from build123d import *
from build123d.topology import SkipClean

# Parameters (mm, degrees)
BOSS_EXTRUDE1_DEPTH      = 3
SKETCH2_W                = 25
SKETCH2_H                = 2
BOSS_EXTRUDE2_DEPTH      = 40
SKETCH3_R                = 0.625
CUT_EXTRUDE1_DEPTH       = 3
SKETCH4_R                = 0.625
CUT_EXTRUDE2_DEPTH       = 3
SKETCH5_W                = 3
SKETCH5_H                = 25
BOSS_EXTRUDE3_DEPTH      = 40
SKETCH7_W                = 19.5
SKETCH7_H                = 75
CUT_EXTRUDE5_DEPTH       = 40
SKETCH10_W               = 25
SKETCH10_H               = 3
BOSS_EXTRUDE4_DEPTH      = 10
SKETCH11_W               = 25
SKETCH11_H               = 3
BOSS_EXTRUDE5_DEPTH      = 10
SKETCH12_W               = 3
SKETCH12_H               = 25
BOSS_EXTRUDE6_DEPTH      = 10
SKETCH13_W               = 3
SKETCH13_H               = 25
BOSS_EXTRUDE7_DEPTH      = 10
SKETCH14_W               = 43
SKETCH14_H               = 35.95813892
BOSS_EXTRUDE11_DEPTH     = 3
SKETCH15_W               = 43
SKETCH15_H               = 35.95813892
BOSS_EXTRUDE12_DEPTH     = 3
SKETCH16_W               = 23
SKETCH16_H               = 28
CUT_EXTRUDE6_DEPTH       = 13
CUT_EXTRUDE7_DEPTH       = 74.054773971
CUT_EXTRUDE7_DEPTH_BACK  = 74.054773971
SKETCH6_R                = 1.625
SKETCH6_R_2              = 3
FILLET1_R                = 10
FILLET2_R                = 10
SKETCH17_W               = 3
SKETCH17_H               = 2.5
CUT_EXTRUDE8_DEPTH       = 30
SKETCH19_W               = 28
SKETCH19_H               = 32
CUT_EXTRUDE9_DEPTH       = 40
CUT_EXTRUDE11_DEPTH      = 60.949979149
CUT_EXTRUDE11_DEPTH_BACK = 60.949979149
SKETCH20_W               = 25.25
SKETCH20_H               = 11.847644437
SKETCH20_W_2             = 25
SKETCH20_H_2             = 13.837487399
CUT_EXTRUDE12_DEPTH      = 70.835521048
CUT_EXTRUDE12_DEPTH_BACK = 70.835521048
CUT_EXTRUDE13_DEPTH      = 56.982140009
CUT_EXTRUDE13_DEPTH_BACK = 56.982140009
SKETCH22_W               = 10
SKETCH22_H               = 25
CUT_EXTRUDE14_DEPTH      = 10
CUT_EXTRUDE14_DEPTH_BACK = 10
SKETCH24_W               = 5.5
SKETCH24_H               = 6.5
SKETCH24_H_2             = 6.525307194


with BuildPart() as part:
    # Sketch1 → Boss-Extrude1 (new body)
    with BuildSketch(Plane.XY):
        Polygon((12.5, 12.5), (21, 12.5), (21, -12.5), (12.5, -12.5), (12.5, -18), (-12.5, -18), (-12.5, -12.5), (-21, -12.5), (-21, 12.5), (-12.5, 12.5), (-12.5, 18), (12.5, 18), align=None)
    extrude(amount=BOSS_EXTRUDE1_DEPTH)

    # Sketch2 → Boss-Extrude2 (add)
    with BuildSketch(Plane.XY.offset(3)):
        with Locations((0, 17)):
            Rectangle(SKETCH2_W, SKETCH2_H)
        with Locations((0, -17)):
            Rectangle(SKETCH2_W, SKETCH2_H)
    extrude(amount=BOSS_EXTRUDE2_DEPTH)

    # Sketch3 → Cut-Extrude1 (cut)
    with BuildSketch(Plane(origin=(0, 18, 0), x_dir=(1, 0, 0), z_dir=(0, 1, 0))):
        with Locations(Location((-11, -17.5, 0), (0, 0, 270))):
            Circle(SKETCH3_R)
        with Locations(Location((11, -17.5, 0), (0, 0, 270))):
            Circle(SKETCH3_R)
        with Locations(Location((-11, -41.5, 0), (0, 0, 270))):
            Circle(SKETCH3_R)
        with Locations(Location((11, -41.5, 0), (0, 0, 270))):
            Circle(SKETCH3_R)
    extrude(amount=-CUT_EXTRUDE1_DEPTH, mode=Mode.SUBTRACT)

    # Sketch4 → Cut-Extrude2 (cut)
    with BuildSketch(Plane(origin=(0, -16, 0), x_dir=(1, 0, 0), z_dir=(0, 1, 0))):
        with Locations(Location((-11, -41.5, 0), (0, 0, 270))):
            Circle(SKETCH4_R)
        with Locations(Location((11, -41.5, 0), (0, 0, 270))):
            Circle(SKETCH4_R)
        with Locations(Location((-11, -21, 0), (0, 0, 270))):
            Circle(SKETCH4_R)
        with Locations(Location((11, -21, 0), (0, 0, 270))):
            Circle(SKETCH4_R)
    extrude(amount=-CUT_EXTRUDE2_DEPTH, mode=Mode.SUBTRACT)

    # Sketch5 → Boss-Extrude3 (add)
    with BuildSketch(Plane(origin=(0, 0, 0), x_dir=(-1, 0, 0), z_dir=(0, 0, -1))):
        with Locations((-19.5, 0)):
            Rectangle(SKETCH5_W, SKETCH5_H)
        with Locations((19.5, 0)):
            Rectangle(SKETCH5_W, SKETCH5_H)
    extrude(amount=BOSS_EXTRUDE3_DEPTH)

    # Sketch7 → Cut-Extrude5 (cut)
    with BuildSketch(Plane(origin=(0, 18, 0), x_dir=(1, 0, 0), z_dir=(0, 1, 0))):
        with Locations((0, -43)):
            Rectangle(SKETCH7_W, SKETCH7_H)
    extrude(amount=-CUT_EXTRUDE5_DEPTH, mode=Mode.SUBTRACT)

    # Sketch10 → Boss-Extrude4 (add)
    with BuildSketch(Plane(origin=(0, 18, 0), x_dir=(1, 0, 0), z_dir=(0, 1, 0))):
        with Locations((0, -1.5)):
            Rectangle(SKETCH10_W, SKETCH10_H)
    extrude(amount=BOSS_EXTRUDE4_DEPTH)

    # Sketch11 → Boss-Extrude5 (add)
    with BuildSketch(Plane.XZ.offset(18)):
        with Locations((0, 1.5)):
            Rectangle(SKETCH11_W, SKETCH11_H)
    extrude(amount=BOSS_EXTRUDE5_DEPTH)

    # Sketch12 → Boss-Extrude6 (add)
    with BuildSketch(Plane.ZY.offset(21)):
        with Locations((1.5, 0)):
            Rectangle(SKETCH12_W, SKETCH12_H)
    extrude(amount=BOSS_EXTRUDE6_DEPTH)

    # Sketch13 → Boss-Extrude7 (add)
    with BuildSketch(Plane(origin=(21, 0, 0), x_dir=(0, 0, -1), z_dir=(1, 0, 0))):
        with Locations((-1.5, 0)):
            Rectangle(SKETCH13_W, SKETCH13_H)
    extrude(amount=BOSS_EXTRUDE7_DEPTH)

    # Sketch14 → Boss-Extrude11 (add)
    with BuildSketch(Plane.ZY.offset(12.5)):
        with Locations((21.5, 0.02093054)):
            Rectangle(SKETCH14_W, SKETCH14_H)
    extrude(amount=BOSS_EXTRUDE11_DEPTH)

    # Sketch15 → Boss-Extrude12 (add)
    with BuildSketch(Plane(origin=(12.5, 0, 0), x_dir=(0, 0, -1), z_dir=(1, 0, 0))):
        with Locations((-21.5, 0.02093054)):
            Rectangle(SKETCH15_W, SKETCH15_H)
    extrude(amount=BOSS_EXTRUDE12_DEPTH)

    # Sketch16 → Cut-Extrude6 (cut)
    with BuildSketch(Plane(origin=(0, 0, 0), x_dir=(-1, 0, 0), z_dir=(0, 0, -1))):
        Rectangle(SKETCH16_W, SKETCH16_H)
    extrude(amount=-CUT_EXTRUDE6_DEPTH, mode=Mode.SUBTRACT)

    # Sketch6 → Cut-Extrude7 (cut, two sides: drawn at the far end of the back side and taken through both)
    with BuildSketch(Plane(origin=(21, 0, 0), x_dir=(0, 0, -1), z_dir=(1, 0, 0)).offset(-CUT_EXTRUDE7_DEPTH_BACK)):
        with Locations(Location((30, 7, 0), (0, 0, 90))):
            Circle(SKETCH6_R)
        with Locations(Location((30, 0, 0), (0, 0, 90))):
            Circle(SKETCH6_R_2)
        with Locations(Location((37, 0, 0), (0, 0, 90))):
            Circle(SKETCH6_R)
        with Locations(Location((30, -7, 0), (0, 0, 90))):
            Circle(SKETCH6_R)
        with Locations(Location((23, 0, 0), (0, 0, 90))):
            Circle(SKETCH6_R)
        with BuildLine():
            Line((30, 10), (30, 12.5))
            Line((30, 12.5), (46.457343261, 12.5))
            Line((46.457343261, 12.5), (46.457343261, -12.5))
            Line((46.457343261, -12.5), (30, -12.5))
            Line((30, -12.5), (30, -10))
            ThreePointArc((30, -10), (40, 0), (30, 10))
        make_face()
    extrude(amount=CUT_EXTRUDE7_DEPTH + CUT_EXTRUDE7_DEPTH_BACK, mode=Mode.SUBTRACT)

    # Fillet1
    fillet1_edges = [part.edges().sort_by_distance(p)[0] for p in [
        (31, 12.5, 1.5),
    ]]
    fillet(fillet1_edges, radius=FILLET1_R)

    # Fillet2
    fillet2_edges = [part.edges().sort_by_distance(p)[0] for p in [
        (12.5, 28, 1.5),
        (-12.5, 28, 1.5),
        (-31, 12.5, 1.5),
        (12.5, -28, 1.5),
        (-31, -12.5, 1.5),
        (-12.5, -28, 1.5),
        (31, -12.5, 1.5),
    ]]
    fillet(fillet2_edges, radius=FILLET2_R - 0.0001)  # a hair under: the kernel refuses the full size

    # Sketch17 → Cut-Extrude8 (cut)
    with BuildSketch(Plane(origin=(0, 0, -30), x_dir=(-1, 0, 0), z_dir=(0, 0, -1))):
        with Locations((-19.5, 11.25)):
            Rectangle(SKETCH17_W, SKETCH17_H)
        with Locations((-19.5, -11.25)):
            Rectangle(SKETCH17_W, SKETCH17_H)
        with Locations((19.5, 11.25)):
            Rectangle(SKETCH17_W, SKETCH17_H)
        with Locations((19.5, -11.25)):
            Rectangle(SKETCH17_W, SKETCH17_H)
    extrude(amount=-CUT_EXTRUDE8_DEPTH, mode=Mode.SUBTRACT)

    # Sketch19 → Cut-Extrude9 (cut)
    with BuildSketch(Plane.XY.offset(43)):
        Rectangle(SKETCH19_W, SKETCH19_H)
    extrude(amount=-CUT_EXTRUDE9_DEPTH, mode=Mode.SUBTRACT)

    # Sketch20 → Cut-Extrude11 (cut, two sides: drawn at the far end of the back side and taken through both)
    with BuildSketch(Plane.XY.offset(3).offset(-CUT_EXTRUDE11_DEPTH_BACK)):
        with Locations((0, 23.923822218)):
            Rectangle(SKETCH20_W, SKETCH20_H)
        with Locations((0, -24.918743699)):
            Rectangle(SKETCH20_W_2, SKETCH20_H_2)
    extrude(amount=CUT_EXTRUDE11_DEPTH + CUT_EXTRUDE11_DEPTH_BACK, mode=Mode.SUBTRACT)

    # Sketch21 → Cut-Extrude12 (cut, two sides: drawn at the far end of the back side and taken through both)
    with SkipClean():  # the faces are left unmerged after this step: merging them gives an invalid solid
        with BuildSketch(Plane.ZY.offset(21).offset(-CUT_EXTRUDE12_DEPTH_BACK)):
            with BuildLine():
                Line((-30, 10), (0, 10))
                Line((0, 10), (0, 6))
                Line((0, 6), (-22, 6))
                ThreePointArc((-22, 6), (-25.527864045, 8.94427191), (-30, 10))
            make_face()
            with BuildLine():
                Line((-22, -6), (0, -6))
                Line((0, -6), (0, -10))
                Line((0, -10), (-30, -10))
                ThreePointArc((-30, -10), (-25.527864045, -8.94427191), (-22, -6))
            make_face()
        extrude(amount=CUT_EXTRUDE12_DEPTH + CUT_EXTRUDE12_DEPTH_BACK, mode=Mode.SUBTRACT)

    # Sketch22 → Cut-Extrude13 (cut, two sides: drawn at the far end of the back side and taken through both)
    with SkipClean():  # the faces are left unmerged after this step: merging them gives an invalid solid
        with BuildSketch(Plane(origin=(0, 0, 0), x_dir=(-1, 0, 0), z_dir=(0, 0, -1)).offset(-CUT_EXTRUDE13_DEPTH_BACK)):
            with Locations((26, 0)):
                Rectangle(SKETCH22_W, SKETCH22_H)
            with Locations((-26, 0)):
                Rectangle(SKETCH22_W, SKETCH22_H)
        extrude(amount=CUT_EXTRUDE13_DEPTH + CUT_EXTRUDE13_DEPTH_BACK, mode=Mode.SUBTRACT)

    # Sketch24 → Cut-Extrude14 (cut, two sides: drawn at the far end of the back side and taken through both)
    with SkipClean():  # the faces are left unmerged after this step: merging them gives an invalid solid
        with BuildSketch(Plane(origin=(0, 0, 0), x_dir=(-1, 0, 0), z_dir=(0, 0, -1)).offset(-CUT_EXTRUDE14_DEPTH_BACK)):
            with Locations((18.25, 9.25)):
                Rectangle(SKETCH24_W, SKETCH24_H)
            with Locations((18.25, -9.237346403)):
                Rectangle(SKETCH24_W, SKETCH24_H_2)
            with Locations((-18.25, -9.237346403)):
                Rectangle(SKETCH24_W, SKETCH24_H_2)
            with Locations((-18.25, 9.25)):
                Rectangle(SKETCH24_W, SKETCH24_H)
        extrude(amount=CUT_EXTRUDE14_DEPTH + CUT_EXTRUDE14_DEPTH_BACK, mode=Mode.SUBTRACT)


solid = part.part
Could you check a few things on this model? Use its own coordinates, in mm. A direction names the side the tool comes from. Give positions to 0.01 mm unless a question says otherwise; leave off trailing zeros. Order: outer loops, then holes, each group sorted by start corner. A loop starts at its lowest first (then second) coordinate and runs counter-clockwise, first axis right, second up.
1. Will these pins go through, and if not, where does the flat tip stop? P1, Ø9, axis at x = 5.5, y = -13.5, coming from the -Z side; P2, Ø3.5, axis at y = 8, z = 1.5, coming from the +X side; P3, Ø8, axis at y = 8.5, z = 28.5, coming from the -X side.
2. For faces 1 (the flat face through (-19, -5.975, -2)), 2 (the flat face through (-13, 0, 3)), 3 (the flat face through (-19, -6, -16)), 4 (the flat face through (9.75, -17, 25)), which set-ups out of +Z, -Z, +X, -X, +Y, -Y let a thin tool reach every point of the face, with its end or its side?
3. Suppose I cut it at C-C (z = 4.5). List the corners of the cut face in (x, y) for me.
4. Suppose I cut it at A-A (x = 8.5). List the corners of the cut face in (y, z) for me, plus the area to 3 significant figures.
5. Suppose I cut it at B-B (z = 24). List the corners of the cut face in (x, y) for me.
6. We'd pull the mould along Z, two halves only. Please class faces 5 (the cylindrical face through (-19.52, -7.21, -28.39)), 6 (the flat face through (-18, 0, -20)), 7 (the flat face through (0, -17, 5.5)): pulls with the +Z half, pulls with the -Z half, needs draft (parallel to the pull), parting line crosses it, or undercut.
7. Suppose I cut it at D-D (z = -37). List the corners of the cut face in (x, y) for me (3 decimals).
8. I need wall thicknesses on L1, parallel to Y at x = 20.05, z = -30 (3 decimals); L2, parallel to X at y = 16.6, z = 41.5 (3 decimals); L3, parallel to X at y = -7, z = 32. Which ranges of each line are inside material? Lowest first, please.
Solved:
1. P1: stops at z = 0
1. P2: stops at x = 15.5
1. P3: stops at x = -15.5
2. face 1: +Z, -X, -Y
2. face 2: +Z
2. face 3: +Z, +X, -X, -Y
2. face 4: +Z, +Y, -Y
3. outline: (-15.5, -17.96) - (-12.5, -17.96) - (-12.5, -18) - (12.5, -18) - (12.5, -17.96) - (15.5, -17.96) - (15.5, 18) - (-15.5, 18) - close; hole (-14, -16) - (14, -16) - (14, 16) - (-14, 16) - close
4. outline: (-18, 0) - (-14, 0) - (-14, 3) - (-16, 3) - (-16, 5.5) - (-18, 5.5) - close; (14, 0) - (18, 0) - (18, 5.5) - (16, 5.5) - (16, 3) - (14, 3) - close
4. area: 34.0 mm2
5. outline: (-15.5, -17.96) - (-12.5, -17.96) - (-12.5, -18) - (-9.75, -18) - (-9.75, -16) - (-14, -16) - (-14, 16) - (-9.75, 16) - (-9.75, 18) - (-15.5, 18) - close; (9.75, -18) - (12.5, -18) - (12.5, -17.96) - (15.5, -17.96) - (15.5, 18) - (9.75, 18) - (9.75, 16) - (14, 16) - (14, -16) - (9.75, -16) - close
6. face 5: undercut
6. face 6: needs draft
6. face 7: pulls with the +Z half
7. outline: (-21, -7.141) - (-18, -7.141) - (-18, -1.625) - (-21, -1.625) - close; (-21, 1.625) - (-18, 1.625) - (-18, 7.141) - (-21, 7.141) - close; (18, -7.141) - (21, -7.141) - (21, -1.625) - (18, -1.625) - close; (18, 1.625) - (21, 1.625) - (21, 7.141) - (18, 7.141) - close
8. L1: y = -10 to -8.625, -5.375 to -3, 3 to 5.375, 8.625 to 10
8. L2: x = -15.5 to -11.625, -10.375 to -9.75, 9.75 to 10.375, 11.625 to 15.5
8. L3: x = -15.5 to -14, 14 to 15.5
